Work out the finished part from the listing and answer in its coordinate system (mm). Face numbers are marked on the shaded views. A direction names the side the tool comes from. Round coordinates to 2 decimals unless told otherwise and drop trailing zeros. Order: outer loops, then holes, each group sorted by start corner. A loop starts at its lowest first (then second) coordinate and runs counter-clockwise, first axis right, second up. Notation, with made-up numbers: (-2.5, 1) - (27.5, 1) arc R15 ccw to (27.5, 28) - close; hole circle Ø6 at (-27, 42). An arc over 180 degrees is marked (long way). Use one line per item in the form item = value. Start each with the question number.
Q1. The part is cut by section A-A on z = 7.25. Determine the outline of the cut face in (x, y), plus the area to 3 significant figures.
Q2. Which of the six approach directions +Z, -Z, +X, -X, +Y, -Y give full straight-line access (tool end or side, diameter ignored) to the marked faces 1, 2, 3, 4 and 5?
Q3. The part is cut by section D-D on z = 5. Determine the outline of the cut face in (x, y), plus the area to 3 significant figures.
Q4. Given P1, Ø0.9, axis at y = -5.5, z = 4, coming from the +X side; P2, Ø1.7, axis at x = 1.5, z = 5, coming from the -Y side; P3, Ø4.5, axis at x = -3, y = -3.5, coming from the -Z side; P4, Ø3, axis at y = 3, z = 5.5, coming from the -X side, each flat-ended and moving along its own axis, determine where each tip first touches the part or whether it passes through.
Q5. Find the intervals of material crossed by line 1 (X direction, y = 1, z = 5); line 2 (X direction, y = -5.75, z = 6.25), in increasing order. Write a range as [from, to].
Q6. The part is cut by section B-B on y = 0.25. Determine the outline of the cut face in (x, z), plus the area to 3 significant figures.
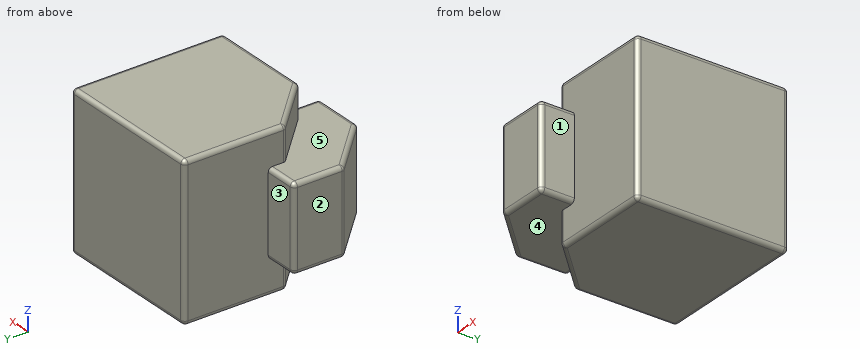
from build123d import *

# Parameters (mm, degrees)
F0_W     = 9
F0_H     = 9
F1_DEPTH = 9
F3_START = 2
F2_W     = 6
F2_H     = 6
F3_DEPTH = 5
F4_SIZE  = 3
F5_SIZE  = 3
F6_SIZE  = 3
F9_R     = 0.25


# Not quite as in the source:
# - a feature of the source that left no trace in its solid (it failed there, or was rolled back) is left out


with BuildPart() as f1:
    # F0 (on Top) → F1 (new body)
    with BuildSketch(Plane.XY):
        Rectangle(F0_W, F0_H)
    extrude(amount=F1_DEPTH)

    # F2 (on Top) → F3 (join)
    with BuildSketch(Plane.XY.offset(F3_START)):
        with Locations((-3.5, -3.5)):
            Rectangle(F2_W, F2_H)
    extrude(amount=F3_DEPTH)

    # F4
    f4_edges = [f1.edges().sort_by_distance(p)[0] for p in [
        (-4.5, -4.5, 1),
    ]]
    chamfer(f4_edges, length=F4_SIZE)

    # F5
    f5_edges = [f1.edges().sort_by_distance(p)[0] for p in [
        (-6.5, -6.5, 4.5),
    ]]
    chamfer(f5_edges, length=F5_SIZE)

    # F6
    f6_edges = [f1.edges().sort_by_distance(p)[0] for p in [
        (-4.5, -4.5, 8),
    ]]
    chamfer(f6_edges, length=F6_SIZE)

    # F9
    f9_edges = [f1.edges().sort_by_distance(p)[0] for p in [
        (-0.5, -6.5, 4.5),
        (-0.5, -5.5, 7),
        (-0.5, -5.5, 2),
        (-2, -6.5, 2),
        (-2, -6.5, 7),
        (-3.5, -6.5, 4.5),
        (-5, -5, 7),
        (-5, -5, 2),
        (-6.5, -3.5, 4.5),
        (-6.5, -2, 7),
        (-6.5, -0.5, 4.5),
        (-6.5, -2, 2),
        (-5.5, -0.5, 2),
        (-5.5, -0.5, 7),
        (-4.5, 1.5, 9),
        (-4.5, -1.5, 8),
        (-4.5, 4.5, 4.5),
        (-4.5, 1.5, 0),
        (-4.5, -1.5, 1),
        (1.5, -4.5, 9),
        (-3, -3, 9),
        (4.5, 0, 9),
        (0, 4.5, 9),
        (-1.5, -4.5, 8),
        (4.5, 4.5, 4.5),
        (0, 4.5, 0),
        (1.5, -4.5, 0),
        (-3, -3, 0),
        (4.5, 0, 0),
        (-1.5, -4.5, 1),
        (4.5, -4.5, 4.5),
    ]]
    fillet(f9_edges, radius=F9_R)


solid = f1.part
Found:
q1.outline = (-4.5, -1.4) arc R0.25 ccw to (-4.43, -1.57) - (-1.57, -4.43) arc R0.25 ccw to (-1.4, -4.5) - (4.25, -4.5) arc R0.25 ccw to (4.5, -4.25) - (4.5, 4.25) arc R0.25 ccw to (4.25, 4.5) - (-4.25, 4.5) arc R0.25 ccw to (-4.5, 4.25) - close
q1.area = 76.5 mm²
q2.face_1 = +Z, -Z, +X, -Y
q2.face_2 = +Z, -Z, -X, +Y, -Y
q2.face_3 = +Z, -Z, -X, +Y
q2.face_4 = -Z, -X, -Y
q2.face_5 = +Z, -X, -Y
q3.outline = (-6.5, -3.4) arc R0.25 ccw to (-6.43, -3.57) - (-3.57, -6.43) arc R0.25 ccw to (-3.4, -6.5) - (-0.75, -6.5) arc R0.25 ccw to (-0.5, -6.25) - (-0.5, -4.5) - (4.25, -4.5) arc R0.25 ccw to (4.5, -4.25) - (4.5, 4.25) arc R0.25 ccw to (4.25, 4.5) - (-4.25, 4.5) arc R0.25 ccw to (-4.5, 4.25) - (-4.5, -0.5) - (-6.25, -0.5) arc R0.25 ccw to (-6.5, -0.75) - close
q3.area = 96.4 mm²
q4.P1 = -0.5
q4.P2 = -4.5
q4.P3 = 0
q4.P4 = -4.5
q5.line_1 = [-4.5, 4.5]
q5.line_2 = [-4.25, -0.5]
q6.outline = (-4.5, 0.25) arc R0.25 ccw to (-4.25, 0) - (4.25, 0) arc R0.25 ccw to (4.5, 0.25) - (4.5, 8.75) arc R0.25 ccw to (4.25, 9) - (-4.25, 9) arc R0.25 ccw to (-4.5, 8.75) - close
q6.area = 80.9 mm²
